Geometry check sheet. Reference: drawing and pictorial views, mm from the part's lowest x, y, z. A direction names the side the tool comes from. Give positions to 0.01 mm unless a question says otherwise; leave off trailing zeros. Order: outer loops, then holes, each group sorted by start corner. A loop starts at its lowest first (then second) coordinate and runs counter-clockwise, first axis right, second up. Notation, with made-up numbers: (-5.75, -3) -> (15.25, -3) arc R36 cw to (15.25, 36) -> close; hole circle Ø5 at (58, 50). An arc over 180 degrees is marked (long way). Write each question's results on one line, items separated by ' | '. Start each with the question number.
1. Cross-section at B-B, the plane x = 5. Enter the section's corners in (y, z) (1 decimal).
2. Depth check by flat-ended pin: pin 1 Ø7 at (x, y) = (6.5, 24) entering from -Z; pin 2 Ø7 at (y, z) = (25, 29.5) entering from -X; pin 3 Ø6 at (y, z) = (13.5, 23.5) entering from -X. Enter the tip coordinate at first touch or a pass-through.
3. Set-up check for the marked faces 1, 2 and 3: record each of +Z, -Z, +X, -X, +Y, -Y from which the full face is reachable in a straight line by a thin tool's end or side.
4. Material ranges on L1, parallel to X at y = 12.5, z = 24 (1 decimal); L2, parallel to X at y = 25.5, z = 28; L3, parallel to Z at x = 67.5, y = 14, recorded low to high. Write a range as from..to.
5. Cross-section at A-A, the plane y = 14.5. Enter the section's corners in (x, z) (1 decimal), then the cut area to 3 significant figures.
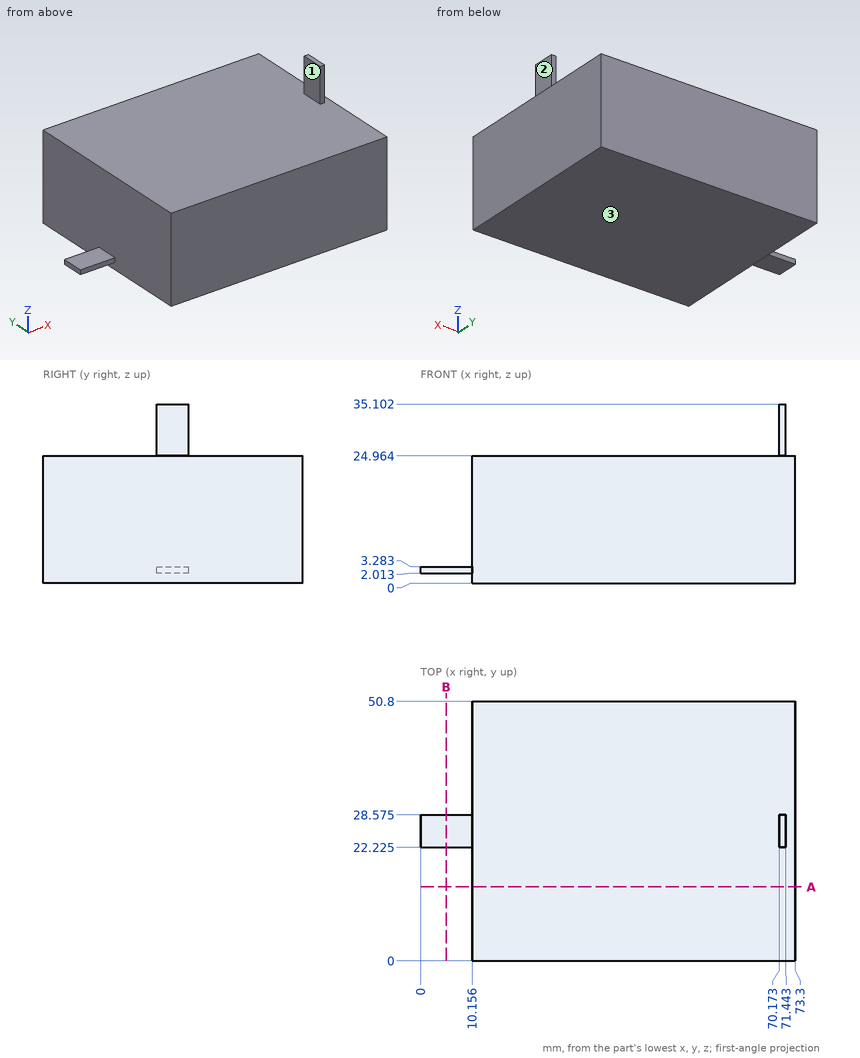
Results below:
1) outline: (22.2, 2) -> (28.6, 2) -> (28.6, 3.3) -> (22.2, 3.3) -> close
2) pin 1: stops at z = 2.01 | pin 2: stops at x = 70.17 | pin 3: stops at x = 10.16
3) face 1: +Z, -X, +Y, -Y | face 2: +Z, +X, +Y, -Y | face 3: -Z, +X, -X, +Y, -Y
4) L1: x = 10.2..73.3 | L2: x = 70.17..71.44 | L3: z = 0..24.96
5) outline: (10.2, 0) -> (73.3, 0) -> (73.3, 25) -> (10.2, 25) -> close | area: 1,580 mm²
